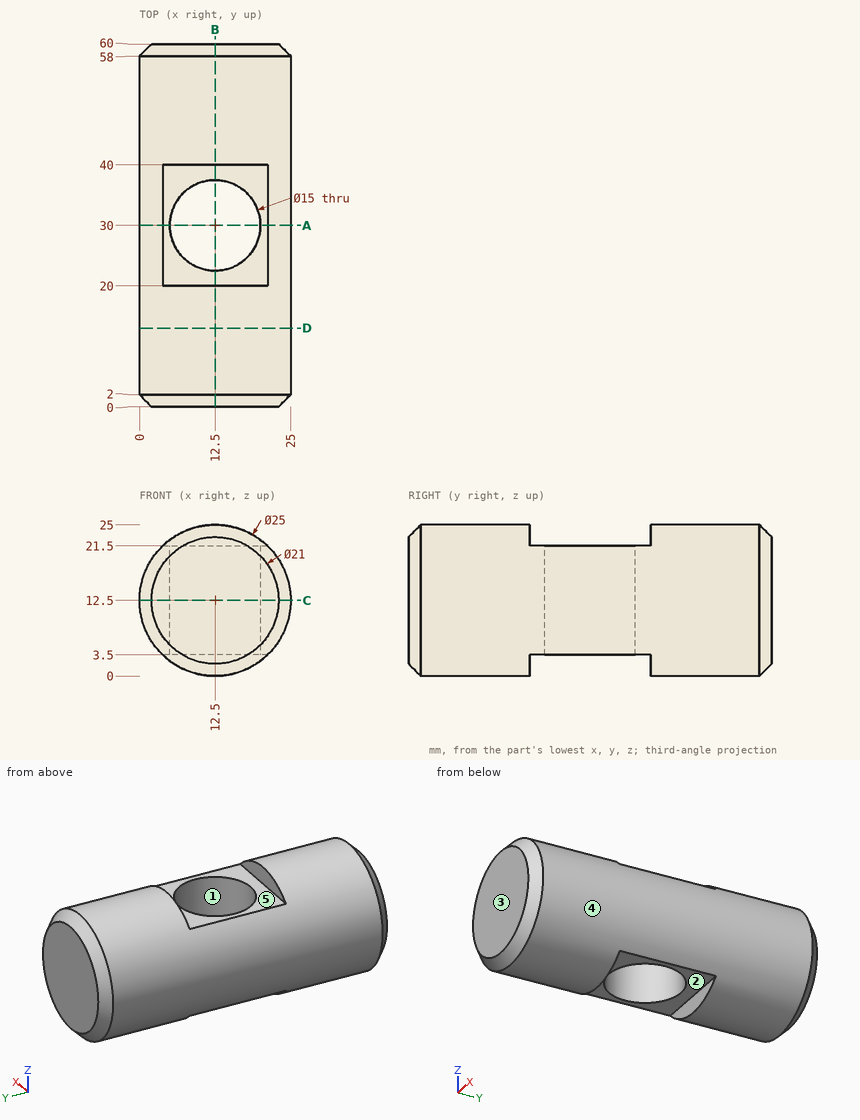
For this review, use the dimensioned drawing (mm, ordinates from the lowest corner) and the shaded views. A direction names the side the tool comes from. Round coordinates to 2 decimals unless told otherwise and drop trailing zeros. Order: outer loops, then holes, each group sorted by start corner. A loop starts at its lowest first (then second) coordinate and runs counter-clockwise, first axis right, second up. Notation, with made-up numbers: (7, -37) -> (34, -37) arc R21 cw to (34, -10) -> close; hole circle Ø3 at (-35, 78.5). An arc over 180 degrees is marked (long way). One line per item, written item: value. Start each with the question number.
Q1. Clearance check with flat-ended pins moving along their axes: pin 1 Ø10 at (x, y) = (19.5, 50) entering from -Z; pin 2 Ø5 at (y, z) = (48.5, 22) entering from +X; pin 3 Ø1.8 at (x, z) = (8.5, 23.5) entering from +Y. State where each tip first meets the part, or that it passes through.
Q2. Machinability: for the marked faces 1 and 2, which of the approach directions +Z, -Z, +X, -X, +Y, -Y give a long, thin tool a straight path to every point of the face, cutting with its end or side? Answer none if there is none.
Q3. Take a section at B-B (x = 12.5). Write out the cut boundary in (y, z).
Q4. Take a section at C-C (z = 12.5). Write out the cut boundary in (x, y).
Q5. Mouldability with a two-part tool opening along Y and no side actions: class the marked faces 3, 4 and 5 as released by +Y, released by -Y, zero draft, split by the parting line, or undercut.
Q6. Take a section at A-A (y = 30). Write out the cut boundary in (x, z), and give its area (3 significant figures).
Q7. Take a section at D-D (y = 13). Write out the cut boundary in (x, z), and give its area (3 significant figures).
Q8. Wall thickness on line 1 (Y direction, x = 12.5, z = 12.5); line 2 (X direction, y = 17, z = 3.5); line 3 (X direction, y = 32, z = 13.5): over which ranges is each line inside the solid? List them lowest first.
Reported:
1. pin 1: stops at z = 0.16
1. pin 2: stops at x = 22.86
1. pin 3: stops at y = 59.7
2. face 1: +Z, -Z
2. face 2: -Z, +X, -X
3. outline: (0, 2) -> (2, 0) -> (20, 0) -> (20, 3.5) -> (22.5, 3.5) -> (22.5, 21.5) -> (20, 21.5) -> (20, 25) -> (2, 25) -> (0, 23) -> close; (37.5, 3.5) -> (40, 3.5) -> (40, 0) -> (58, 0) -> (60, 2) -> (60, 23) -> (58, 25) -> (40, 25) -> (40, 21.5) -> (37.5, 21.5) -> close
4. outline: (0, 2) -> (2, 0) -> (23, 0) -> (25, 2) -> (25, 58) -> (23, 60) -> (2, 60) -> (0, 58) -> close; hole circle Ø15 at (12.5, 30)
5. face 3: released by -Y
5. face 4: zero draft
5. face 5: undercut
6. outline: (3.83, 3.5) -> (5, 3.5) -> (5, 21.5) -> (3.83, 21.5) arc R12.5 ccw to start; (20, 3.5) -> (21.17, 3.5) arc R12.5 ccw to (21.17, 21.5) -> (20, 21.5) -> close
6. area: 137 mm2
7. outline: circle Ø25 at (12.5, 12.5)
7. area: 491 mm2
8. line 1: y = 0 to 22.5, 37.5 to 60
8. line 2: x = 3.83 to 21.17
8. line 3: x = 0.04 to 5.27, 19.73 to 24.96
